Design review of the part built by this model. Coordinates are the model's own, in mm. Face numbers are marked on the shaded views. A direction names the side the tool comes from. Give positions to 0.01 mm unless a question says otherwise; leave off trailing zeros. Loops run counter-clockwise (first coordinate to the right, second up) from the corner with the lowest first, then second, coordinate; pieces in that order, holes last. Notation, with made-up numbers: M 81.5,70 L 109.5,70 A16 cw 109.5,88 Z; hole C 4.5,-2 d6. An arc over 180 degrees is marked long. Use a Markdown table: item, result. Add a question column.
(1) Add section B-B, the plane z = 0. Give the boundary of the cut face in (x, y) (3 decimals).
(2) For the marked faces 4, 5 and 6, list the 3-axis set-ups (+Z, -Z, +X, -X, +Y, -Y) from which the entire face can be reached by the end or side of a thin tool; tool diameter is ignored.
(3) Draft analysis for pull direction Y (two halves, no side actions). For the marked faces 1, 2 and 3, state which applies: pulls with the +Y half, pulls with the -Y half, needs draft (parallel to the pull), parting line crosses it, or undercut.
(4) Add section D-D, the plane z = -5.5. Give the boundary of the cut face in (x, y).
(5) Insertion check: pin 1 Ø1.5 at (y, z) = (-5.93, 5.78) entering from +X. The pin has a flat end and moves straight along its axis. Give the tip position at first contact, or say it passes through.
(6) Add section C-C, the plane x = -1.7. Give the boundary of the cut face in (y, z) (3 decimals).
(7) For probe 1 along Z at (x, y) = (-0.85, -5.5); probe 2 along Y at (x, z) = (0.3, 0.25); probe 3 along X at (y, z) = (4.25, -6), list the stretches that pass through material, from the lowest coordinate up.
(8) Add section A-A, the plane y = 0. Give the boundary of the cut face in (x, z) (3 decimals), then the cut area to 3 significant figures.
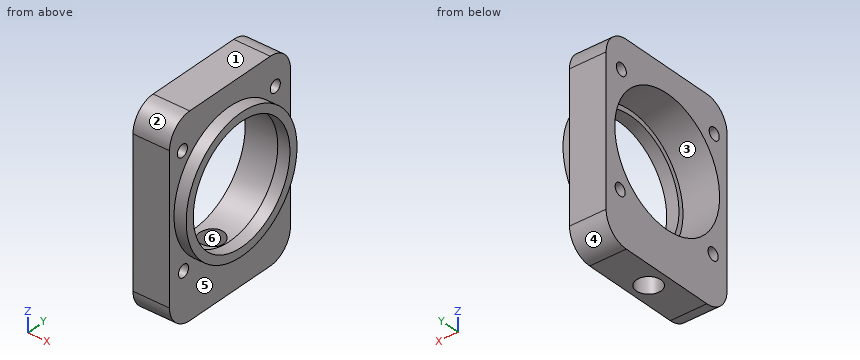
```python
from build123d import *

# Parameters (mm, degrees)
F0_R     = 6.985
F0_R_2   = 6.096
F1_DEPTH = 1.27
F2_R     = 6.604
F3_DEPTH = 3.81
F5_D     = 1.27
F7_D     = 2.54
F7_DEPTH = 5.08
F7_TIP   = 0.7630929862


# Not quite as in the source:
# - a feature names something its author has since deleted; it is built from what else it names


with BuildPart() as f1:
    # F0 (on Right) → F1 (new body)
    with BuildSketch(Plane.YZ):
        Circle(F0_R)
        Circle(F0_R_2, mode=Mode.SUBTRACT)
    extrude(amount=F1_DEPTH)

    # F2 (on Right) → F3 (join)
    with BuildSketch(Plane.YZ):
        with BuildLine():
            Line((5.1588201895, 9.1668736476), (-5.0011798105, 9.1668736476))
            ThreePointArc((-5.0011798105, 9.1668736476), (-6.7972310347, 8.4229248718), (-7.5411798105, 6.6268736476))
            Line((-7.5411798105, 6.6268736476), (-7.5411798105, -8.6131263524))
            ThreePointArc((-7.5411798105, -8.6131263524), (-6.7972310347, -10.4091775766), (-5.0011798105, -11.1531263524))
            Line((-5.0011798105, -11.1531263524), (5.1588201895, -11.1531263524))
            ThreePointArc((5.1588201895, -11.1531263524), (6.9548714137, -10.4091775766), (7.6988201895, -8.6131263524))
            Line((7.6988201895, -8.6131263524), (7.6988201895, 6.6268736476))
            ThreePointArc((7.6988201895, 6.6268736476), (6.9548714137, 8.4229248718), (5.1588201895, 9.1668736476))
        make_face()
        Circle(F2_R, mode=Mode.SUBTRACT)
    extrude(amount=-F3_DEPTH)

    # F5 (through all)
    with Locations(Plane(origin=(-3.81, 0, 0), x_dir=(0, -1, 0), z_dir=(-1, 0, 0))):
        with Locations((5.9254106074, 5.7839893926), (-5.7839893926, 5.9254106074), (5.7839893926, -5.9254106074), (-5.9254106074, -5.7839893926)):
            Hole(F5_D / 2)

    # F7
    with Locations(Plane(origin=(0, 0, -11.1531263524), x_dir=(1, 0, 0), z_dir=(0, 0, -1))):
        with Locations((-1.8845667364, 0)):
            Hole(F7_D / 2, depth=F7_DEPTH)
            with Locations((0, 0, -(F7_DEPTH + F7_TIP / 2))):  # 118° drill point
                Cone(0, F7_D / 2, F7_TIP, mode=Mode.SUBTRACT)


solid = f1.part
```
Established:
| question | item | result |
|---|---|---|
| 1 | outline | M -3.81,-7.541 L 0,-7.541 L 0,-6.985 L 1.27,-6.985 L 1.27,-6.096 L 0,-6.096 L 0,-6.604 L -3.81,-6.604 Z; M -3.81,6.604 L 0,6.604 L 0,6.096 L 1.27,6.096 L 1.27,6.985 L 0,6.985 L 0,7.699 L -3.81,7.699 Z |
| 2 | face 4 | -Z, +X, -X, +Y |
| 2 | face 5 | +X |
| 2 | face 6 | -Z |
| 3 | face 1 | needs draft |
| 3 | face 2 | pulls with the -Y half |
| 3 | face 3 | undercut |
| 4 | outline | M -3.81,-7.54 L 0,-7.54 L 0,-6.26 L -3.81,-6.26 Z; M -3.81,-5.31 L 0,-5.31 L 0,-4.31 L 1.27,-4.31 L 1.27,-2.63 L 0,-2.63 L 0,-3.66 L -3.81,-3.66 Z; M -3.81,3.66 L 0,3.66 L 0,2.63 L 1.27,2.63 L 1.27,4.31 L 0,4.31 L 0,5.36 L -3.81,5.36 Z; M -3.81,6.49 L 0,6.49 L 0,7.7 L -3.81,7.7 Z |
| 5 | pin 1 | x = 0 |
| 6 | outline | M -7.541,-8.613 A2.54 ccw -5.001,-11.153 L -1.257,-11.153 L -1.257,-6.483 A6.604 cw long 1.257,-6.483 L 1.257,-11.153 L 5.159,-11.153 A2.54 ccw 7.699,-8.613 L 7.699,6.627 A2.54 ccw 5.159,9.167 L -5.001,9.167 A2.54 ccw -7.541,6.627 Z; hole C -5.925,5.784 d1.27; hole C -5.784,-5.925 d1.27; hole C 5.784,5.925 d1.27; hole C 5.925,-5.784 d1.27 |
| 7 | probe 1 | -11.1 to -6.49, -5.36 to -3.66, 3.66 to 5.31, 6.26 to 9.12 |
| 7 | probe 2 | -6.98 to -6.09, 6.09 to 6.98 |
| 7 | probe 3 | -3.81 to 0 |
| 8 | outline | M -3.81,-11.153 L -3.155,-11.153 L -3.155,-6.604 L -3.81,-6.604 Z; M -3.81,6.604 L 0,6.604 L 0,6.096 L 1.27,6.096 L 1.27,6.985 L 0,6.985 L 0,9.167 L -3.81,9.167 Z; M -0.615,-11.153 L 0,-11.153 L 0,-6.985 L 1.27,-6.985 L 1.27,-6.096 L 0,-6.096 L 0,-6.604 L -0.615,-6.604 Z |
| 8 | area | 17.8 mm^2 |
